Verification items for the finished model (mm, model axes). A direction names the side the tool comes from. Give positions to 0.01 mm unless a question says otherwise; leave off trailing zeros. Write each loop counter-clockwise with the first axis right and the second up, starting at its lowest first coordinate (ties: lowest second). Pieces come first, ordered by that corner, then holes. Notation, with made-up numbers: (-10.5, 52) - (6.5, 52) arc R13 ccw to (6.5, 63) - close; hole circle Ø10 at (73.5, 70.5). An arc over 180 degrees is marked (long way). Answer as a JSON object with one key per item and string values. Group by question number.
Item 1: Draft check along Z on faces 1 (the face through (13, -10, 12.7)), 2 (the face through (5, -12.7, 6)), 3 (the face through (13, -15, 3.734)). Enter one of: +Z half, -Z half, draft (parallel to the pull), parting line (faces both ways), or undercut.
Item 2: Scan lines: line 1 along Z through (x, y) = (16.75, -16.75); line 2 along Z through (x, y) = (3.25, -4.75); line 3 along X through (y, z) = (-19.05, 11.85). Record each from-to range of solid material in increasing order. Write a range as [from, to].
Item 3: Sectioned sample at B-B, the plane y = -14.25. Record the boundary of the cut face in (x, z), and give its area (3 significant figures).
Item 4: Sectioned sample at D-D, the plane x = 3.25. Record the boundary of the cut face in (y, z).
Item 5: Sectioned sample at C-C, the plane y = -4.25. Count the separate pieces of the cut face and the enclosed holes in it, and give its area (3 significant figures).
Item 6: Go/stop test with flat-tipped pins: pin 1 (1.9 mm diameter, centred on y = -16.5, z = 2.5, fed in from -X); pin 2 (3 mm diameter, centred on y = -16, z = 11, fed in from +X); pin 3 (4 mm diameter, centred on x = 13, z = 6.5, fed in from -Y); pin 4 (4 mm diameter, centred on x = 13.09, y = -19.05, fed in from +Z). Record where each tip stops, or that it passes through.
Item 7: Sectioned sample at A-A, the plane z = 6.35. Record the boundary of the cut face in (x, y), and give its area (3 significant figures).
Item 8: Tool access check on faces 4 (the face through (13, -15, 8.992)), 5 (the face through (19.444, -16, 2)), 6 (the face through (11.306, -1.177, 9.134)), 7 (the face through (6.744, -16, 2)). Record the directions out of +Z, -Z, +X, -X, +Y, -Y that give a thin tool (end or side, any length) a straight path to the whole face; none if there is none.
```python
from build123d import *

# Parameters (mm, degrees)
F0_R     = 3.175
F1_DEPTH = 12.7
F2_R     = 1.5875
F3_DEPTH = 25.401
F4_R     = 3.302
F5_DEPTH = 2.3876
F6_W     = 12.7
F6_H     = 5.2578
F7_DEPTH = 12.701
F8_DEPTH = 1.5748


with BuildPart() as f1:
    # F0 (on Top) → F1 (new body)
    with BuildSketch(Plane.XY):
        with BuildLine():
            Line((26.1874, 0), (0, 0))
            Line((0, 0), (0, -12.7))
            Line((0, -12.7), (6.7437, -12.7))
            Line((6.7437, -12.7), (6.7437, -19.05))
            ThreePointArc((6.7437, -19.05), (13.0937, -25.4), (19.4437, -19.05))
            Line((19.4437, -19.05), (19.4437, -12.7))
            Line((19.4437, -12.7), (26.1874, -12.7))
            Line((26.1874, -12.7), (26.1874, 0))
        make_face()
        with Locations((13.0937, -19.05)):
            Circle(F0_R, mode=Mode.SUBTRACT)
    extrude(amount=F1_DEPTH)

    # F2 (on face) → F3 (cut, through all)
    with BuildSketch(Plane(origin=(0, 0, 0), x_dir=(-1, 0, 0), z_dir=(0, 1, 0))):
        with Locations((-3.175, 6.35)):
            Circle(F2_R)
        with Locations((-23.0124, 6.35)):
            Circle(F2_R)
    extrude(amount=-F3_DEPTH, mode=Mode.SUBTRACT)

    # F4 (on face) → F5 (cut)
    with BuildSketch(Plane(origin=(0, 0, 0), x_dir=(-1, 0, 0), z_dir=(0, 1, 0))):
        with Locations((-13.081, 6.35)):
            Circle(F4_R)
    extrude(amount=-F5_DEPTH, mode=Mode.SUBTRACT)

    # F6 (on face) → F7 (cut, through all)
    with BuildSketch(Plane.XZ.offset(12.7)):
        with Locations((13.0937, 6.3627)):
            Rectangle(F6_W, F6_H)
    extrude(amount=F7_DEPTH, mode=Mode.SUBTRACT)

    # F6 (on face) → F8 (cut)
    with BuildSketch(Plane.XZ.offset(12.7)):
        with Locations((13.0937, 6.3627)):
            Rectangle(F6_W, F6_H)
    extrude(amount=-F8_DEPTH, mode=Mode.SUBTRACT)


solid = f1.part
```
Geometry check:
{
 "1": {"face 1": "+Z half", "face 2": "draft", "face 3": "undercut"},
 "2": {"line 1": "[0, 3.73], [8.99, 12.7]", "line 2": "[0, 4.76], [7.94, 12.7]", "line 3": "[6.74, 9.92], [16.27, 19.44]"},
 "3": {"outline": "(6.74, 0) - (19.44, 0) - (19.44, 3.73) - (6.74, 3.73) - close; (6.74, 8.99) - (19.44, 8.99) - (19.44, 12.7) - (6.74, 12.7) - close", "area": "94.5 mm^2"},
 "4": {"outline": "(-12.7, 0) - (0, 0) - (0, 4.76) - (-12.7, 4.76) - close; (-12.7, 7.94) - (0, 7.94) - (0, 12.7) - (-12.7, 12.7) - close"},
 "5": {"separate pieces": "1", "enclosed holes": "2", "area": "317 mm^2"},
 "6": {"pin 1": "x = 6.74", "pin 2": "x = 19.44", "pin 3": "y = -11.13", "pin 4": "through"},
 "7": {"outline": "(0, -12.7) - (1.59, -12.7) - (1.59, 0) - (0, 0) - close; (4.76, -12.7) - (6.74, -12.7) - (6.74, -11.13) - (19.44, -11.13) - (19.44, -12.7) - (21.42, -12.7) - (21.42, 0) - (16.38, 0) - (16.38, -2.39) - (9.78, -2.39) - (9.78, 0) - (4.76, 0) - close; (24.6, -12.7) - (26.19, -12.7) - (26.19, 0) - (24.6, 0) - close", "area": "216 mm^2"},
 "8": {"face 4": "-Y", "face 5": "+Z, -Z, +X, -Y", "face 6": "+Y", "face 7": "+Z, -Z, -X, -Y"}
}
